Design review of the part built by this model. Coordinates are the model's own, in mm. Face numbers are marked on the shaded views. Give positions to 0.01 mm unless a question says otherwise; leave off trailing zeros. Loops run counter-clockwise (first coordinate to the right, second up) from the corner with the lowest first, then second, coordinate; pieces in that order, holes last. Notation, with made-up numbers: (87.5, 72) - (115.5, 72) arc R17 ccw to (115.5, 85) - close; hole circle Ø8 at (-22.5, 77.25). An arc over 180 degrees is marked (long way). One line per item, written item: value. Start each with the question number.
```python
from build123d import *

# Parameters (mm, degrees)
F0_R     = 65
F0_R_2   = 22.5
F1_DEPTH = 55
F2_R     = 5


with BuildPart() as f1:
    # F0 (on Right) → F1 (new body)
    with BuildSketch(Plane.YZ):
        Circle(F0_R)
        Circle(F0_R_2, mode=Mode.SUBTRACT)
    extrude(amount=F1_DEPTH)

    # F2
    f2_edges = [f1.edges().sort_by_distance(p)[0] for p in [
        (27.5, 65, 0),
        (0, -65, 0),
        (55, -65, 0),
        (27.5, 22.5, 0),
        (0, -22.5, 0),
        (55, -22.5, 0),
    ]]
    fillet(f2_edges, radius=F2_R)


solid = f1.part
```
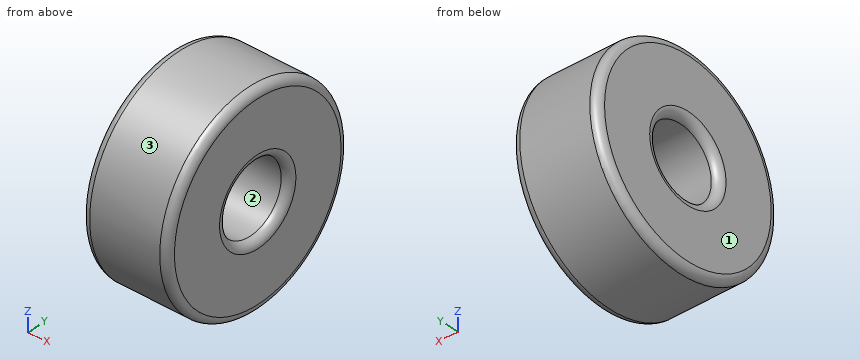
(1) Draft analysis for pull direction Y (two halves, no side actions). For the marked faces 1, 2 and 3, state which applies: pulls with the +Y half, pulls with the -Y half, needs draft (parallel to the pull), parting line crosses it, or undercut.
(2) Take a section at A-A on y = 0. State the section outline as (x, z) points.
(3) For pin 1 Ø10 at (x, z) = (37, 34) entering from -Y; pin 2 Ø6 at (x, y) = (20.5, 3) entering from +Z; pin 3 Ø2 at (y, z) = (-2, 25) entering from +X, all flat-tipped, find the tip position at first contact; note any pin that passes through.
(4) To check wall thickness, follow L1, parallel to Z at x = 33, y = 0; L2, parallel to Y at x = 21, z = -17; L3, parallel to Z at x = 27, y = 2. State the ranges of each line that lie inside material, in increasing order. Write a range as from..to.
(5) Take a section at C-C on x = 21.5. State the section outline as (y, z) points.
Here are the results:
1. face 1: needs draft
1. face 2: undercut
1. face 3: parting line crosses it
2. outline: (0, -60) arc R5 ccw to (5, -65) - (50, -65) arc R5 ccw to (55, -60) - (55, -27.5) arc R5 ccw to (50, -22.5) - (5, -22.5) arc R5 ccw to (0, -27.5) - close; (0, 27.5) arc R5 ccw to (5, 22.5) - (50, 22.5) arc R5 ccw to (55, 27.5) - (55, 60) arc R5 ccw to (50, 65) - (5, 65) arc R5 ccw to (0, 60) - close
3. pin 1: y = -58.17
3. pin 2: z = 65
3. pin 3: x = 54.79
4. L1: -65..-22.5, 22.5..65
4. L2: -62.74..-14.74, 14.74..62.74
4. L3: -64.97..-22.41, 22.41..64.97
5. outline: circle Ø130 at (0, 0); hole circle Ø45 at (0, 0)
